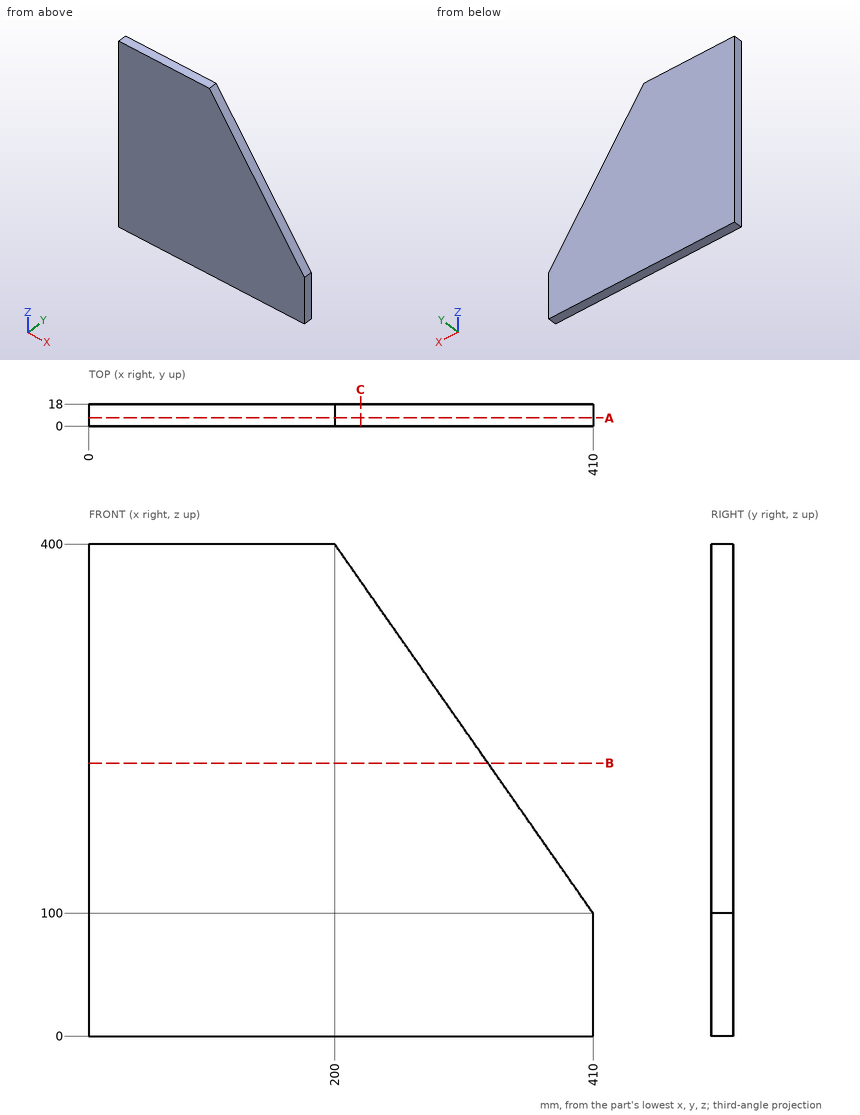
Design review of the part shown in the three views and the two pictorial views. Dimensions are in mm from the part's minimum x, y and z. Round coordinates to 2 decimals unless told otherwise and drop trailing zeros. Loops run counter-clockwise (first coordinate to the right, second up) from the corner with the lowest first, then second, coordinate; pieces in that order, holes last. Notation, with made-up numbers: M -18.5,63.5 L -10.5,63.5 A19 ccw -10.5,84.5 Z; hole C 86.5,52 d9. An arc over 180 degrees is marked long. Write item = value, one per line.
Item 1: Insertion check: P1, Ø3, axis at x = 300, y = 6.5, coming from the +Z side. The pin has a flat end and moves straight along its axis. Give the tip position at first contact, or say it passes through.
Return value:
P1 = 259.29
Item 2: Take a section at A-A on y = 6.75. Write out the cut boundary in (x, z), then the cut area to 4 significant figures.
Return value:
outline = M 0,0 L 410,0 L 410,100 L 200,400 L 0,400 Z
area = 132,500 mm2
Item 3: Take a section at B-B on z = 222. Write out the cut boundary in (x, y).
Return value:
outline = M 0,0 L 324.6,0 L 324.6,18 L 0,18 Z
Item 4: Take a section at C-C on x = 221. Write out the cut boundary in (y, z).
Return value:
outline = M 0,0 L 18,0 L 18,370 L 0,370 Z
Item 5: For line 1 (Z direction, x = 311, y = 14); line 2 (Z direction, x = 203, y = 1); line 3 (X direction, y = 16.5, z = 266), list the stretches that pass through material, from the lowest coordinate up. Write a range as [from, to].
Return value:
line_1 = [0, 241.43]
line_2 = [0, 395.71]
line_3 = [0, 293.8]
